Verification items for the finished model (mm, model axes). Face numbers are marked on the shaded views. Round coordinates to 2 decimals unless told otherwise and drop trailing zeros. Loops run counter-clockwise (first coordinate to the right, second up) from the corner with the lowest first, then second, coordinate; pieces in that order, holes last.
from build123d import *

# Parameters (mm, degrees)
SKETCH_1_R          = 55
EXTRUDE_1_DEPTH     = 80
SKETCH_2_R          = 50
CUT_EXTRUDE_1_DEPTH = 75
SKETCH_3_W          = 33.5
SKETCH_3_H          = 15
CUT_EXTRUDE_2_DEPTH = 6
SKETCH_4_R          = 4
CUT_EXTRUDE_3_DEPTH = 81
SKETCH2_W           = 33.5
SKETCH2_H           = 15
BOSS_EXTRUDE1_DEPTH = 5


with BuildPart() as part:
    # Эскиз1 → Бобышка-Вытянуть1 (new body)
    with BuildSketch(Plane(origin=(0, 0, 0), x_dir=(1, 0, 0), z_dir=(0, 1, 0))):
        Circle(SKETCH_1_R)
    extrude(amount=EXTRUDE_1_DEPTH)

    # Эскиз2 → Вырез-Вытянуть1 (cut)
    with BuildSketch(Plane.XZ):
        Circle(SKETCH_2_R)
    extrude(amount=-CUT_EXTRUDE_1_DEPTH, mode=Mode.SUBTRACT)

    # Эскиз3 → Вырез-Вытянуть2 (cut, through all)
    with BuildSketch(Plane.XZ.offset(-75)):
        Rectangle(SKETCH_3_W, SKETCH_3_H)
    extrude(amount=-CUT_EXTRUDE_2_DEPTH, mode=Mode.SUBTRACT)

    # Эскиз4 → Вырез-Вытянуть3 (cut, through all)
    with BuildSketch(Plane(origin=(0, 80, 0), x_dir=(1, 0, 0), z_dir=(0, 1, 0))):
        with Locations((33.591727056, -32.872418125)):
            Circle(SKETCH_4_R)
        with Locations((-33.591727056, -32.872418125)):
            Circle(SKETCH_4_R)
        with Locations((-33.591727056, 32.872418125)):
            Circle(SKETCH_4_R)
        with Locations((33.591727056, 32.872418125)):
            Circle(SKETCH_4_R)
    extrude(amount=-CUT_EXTRUDE_3_DEPTH, mode=Mode.SUBTRACT)

    # Sketch2 → Boss-Extrude1 (add)
    with BuildSketch(Plane(origin=(0, 80, 0), x_dir=(1, 0, 0), z_dir=(0, 1, 0))):
        Rectangle(SKETCH2_W, SKETCH2_H)
    extrude(amount=-BOSS_EXTRUDE1_DEPTH)


solid = part.part
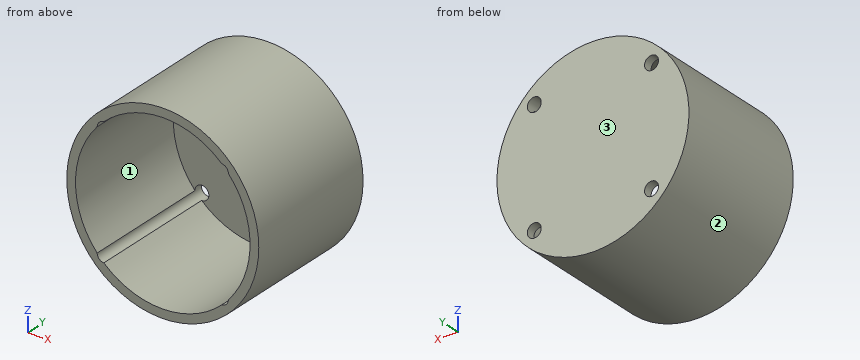
1. Gauge pin test, flat ends, axial feed: P1, Ø6, axis at x = -40.5, y = 56, coming from the -Z side; P2, Ø6.5, axis at x = 33.59, z = -32.87, coming from the +Y side; P3, Ø1.5, axis at x = -43, z = -25, coming from the -Y side; P4, Ø1, axis at x = 38, y = 31, coming from the +Z side. Record the tip position at first contact, or that the pin passes through.
2. Section check B-B (x = 0). Enter the section's corners in (y, z), then the cut area to 3 significant figures.
3. Section check C-C (z = -43). Enter the section's corners in (x, y).
4. Scan lines: L1, parallel to Z at x = -1.5, y = 51; L2, parallel to Y at x = -21.5, z = -37.5; L3, parallel to X at y = 53, z = 31. Record each from-to range of solid material in increasing order.
5. Release check for a two-part mould opening along X. For the marked faces 1, 2 and 3 record: released by +X, released by -X, zero draft, split by the parting line, or undercut.
6. Section check A-A (y = 64.5). Enter the section's corners in (x, z).
Taken from the geometry:
1. P1: stops at z = -40.23
1. P2: passes through
1. P3: stops at y = 0
1. P4: stops at z = 40.23
2. outline: (0, -55) - (80, -55) - (80, 55) - (0, 55) - (0, 50) - (75, 50) - (75, -50) - (0, -50) - close
2. area: 1,300 mm2
3. outline: (-34.29, 0) - (-25.51, 0) - (-25.51, 75) - (25.51, 75) - (25.51, 0) - (34.29, 0) - (34.29, 80) - (-34.29, 80) - close
4. L1: z = -54.98 to -49.98, 49.98 to 54.98
4. L2: y = 75 to 80
4. L3: x = -45.43 to -39.23, 39.23 to 45.43
5. face 1: undercut
5. face 2: split by the parting line
5. face 3: zero draft
6. outline: circle Ø110 at (0, 0); hole (-37.59, -32.97) arc R4 ccw to (-33.77, -36.87) arc R50 ccw to (33.77, -36.87) arc R4 ccw to (37.59, -32.97) arc R50 ccw to (37.59, 32.97) arc R4 ccw to (33.77, 36.87) arc R50 ccw to (-33.77, 36.87) arc R4 ccw to (-37.59, 32.97) arc R50 ccw to start
